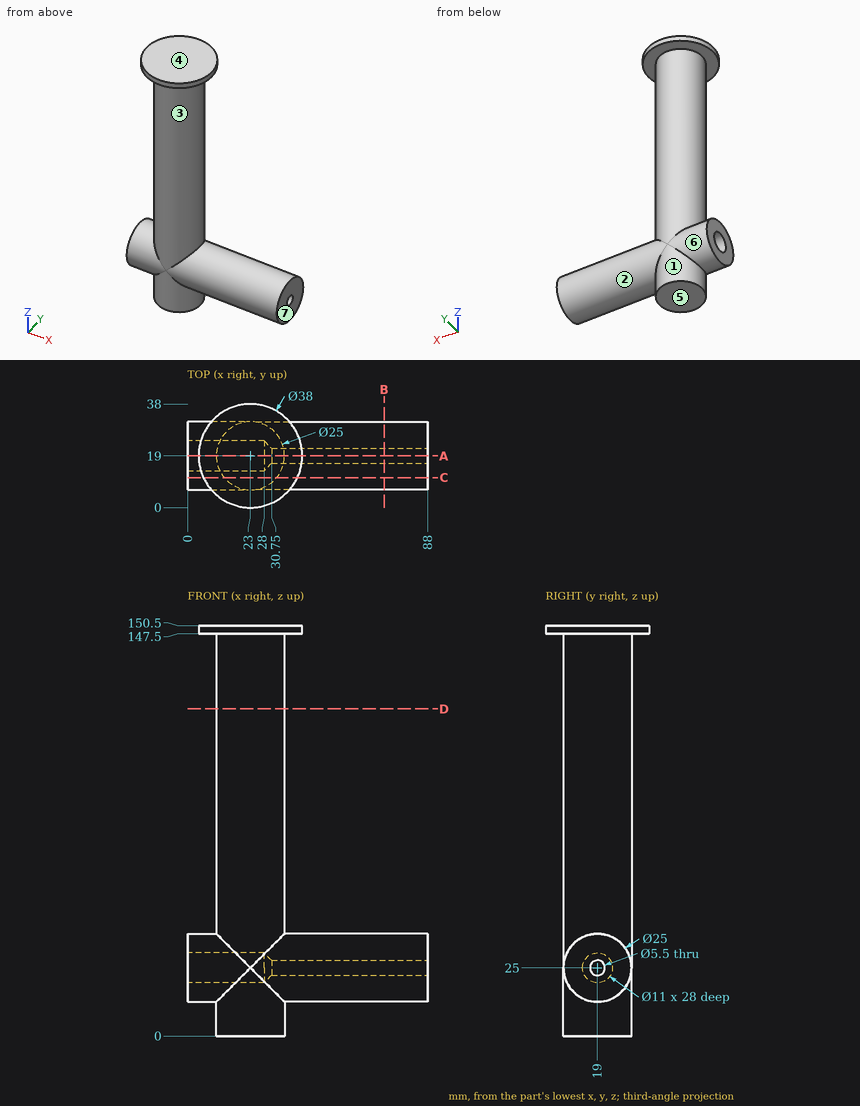
Design review of the part shown in the three views and the two pictorial views. Dimensions are in mm from the part's minimum x, y and z. A direction names the side the tool comes from. Round coordinates to 2 decimals unless told otherwise and drop trailing zeros. Loops run counter-clockwise (first coordinate to the right, second up) from the corner with the lowest first, then second, coordinate; pieces in that order, holes last. Notation, with made-up numbers: M -33.5,-0.75 L 0.5,-0.75 A10 ccw 0.5,15.25 Z; hole C 3.25,88 d8. An arc over 180 degrees is marked long. Answer as a JSON object with one key per item and string values.
Item 1: Wall thickness on L1, parallel to Z at x = 64, y = 19; L2, parallel to Z at x = 32.5, y = 21.5; L3, parallel to Y at x = 22, z = 19: over which ranges is each line inside the solid? List them lowest first. Write a range as from..to.
Answer sheet:
{"L1": "z = 12.5..22.25, 27.75..37.5", "L2": "z = 0..23.85, 26.15..150.5", "L3": "y = 6.54..31.46"}
Item 2: We need section A-A on y = 19. Give the boundary of the cut face in (x, z).
Answer sheet:
{"outline": "M 0,12.5 L 10.5,12.5 L 10.5,0 L 35.5,0 L 35.5,12.5 L 88,12.5 L 88,22.25 L 30.75,22.25 L 28,19.5 L 0,19.5 Z; M 0,30.5 L 28,30.5 L 30.75,27.75 L 88,27.75 L 88,37.5 L 35.5,37.5 L 35.5,147.5 L 42,147.5 L 42,150.5 L 4,150.5 L 4,147.5 L 10.5,147.5 L 10.5,37.5 L 0,37.5 Z"}
Item 3: Clearance check with flat-ended pins moving along their axes: P1, Ø6.5, axis at y = 19, z = 25, coming from the -X side; P2, Ø5, axis at y = 7, z = 49, coming from the -X side; P3, Ø1, axis at x = 36, y = 11.5, coming from the -Z side. State where each tip first meets the part, or that it passes through.
Answer sheet:
{"P1": "stops at x = 30.25", "P2": "stops at x = 14.88", "P3": "stops at z = 14.64"}
Item 4: We need section C-C on y = 11. Give the boundary of the cut face in (x, z), and give its area (3 significant figures).
Answer sheet:
{"outline": "M 0,15.4 L 13.4,15.4 L 13.4,0 L 32.6,0 L 32.6,15.4 L 88,15.4 L 88,34.6 L 32.6,34.6 L 32.6,147.5 L 40.23,147.5 L 40.23,150.5 L 5.77,150.5 L 5.77,147.5 L 13.4,147.5 L 13.4,34.6 L 0,34.6 Z", "area": "4,260 mm^2"}
Item 5: The part is to be moulded in two halves that separate along Z. For the marked faces 4, 5, 6 and 7, say which applies: pulls with the +Z half, pulls with the -Z half, needs draft (parallel to the pull), parting line crosses it, or undercut.
Answer sheet:
{"face 4": "pulls with the +Z half", "face 5": "pulls with the -Z half", "face 6": "undercut", "face 7": "needs draft"}
Item 6: We need section B-B on x = 72. Give the boundary of the cut face in (y, z), and give its area (3 significant figures).
Answer sheet:
{"outline": "C 19,25 d25; hole C 19,25 d5.5", "area": "467 mm^2"}
Item 7: We need section D-D on z = 120. Give the boundary of the cut face in (x, y).
Answer sheet:
{"outline": "C 23,19 d25"}
Item 8: Machinability: for the marked faces 1, 2 and 3, which of the approach directions +Z, -Z, +X, -X, +Y, -Y give a long, thin tool a straight path to every point of the face, cutting with its end or side? Answer none if there is none.
Answer sheet:
{"face 1": "-Z", "face 2": "+X", "face 3": "none"}
